Here's how the part is built. I have some questions about the finished solid (model axes, mm). A direction names the side the tool comes from. Round coordinates to 2 decimals unless told otherwise and drop trailing zeros. Write each loop counter-clockwise with the first axis right and the second up, starting at its lowest first coordinate (ties: lowest second). Pieces come first, ordered by that corner, then holes. Notation, with made-up numbers: (5, 21) -> (42, 21) arc R20 ccw to (42, 27) -> close; hole circle Ø9 at (-5.75, 65.25). An arc over 180 degrees is marked (long way). Put each result on its own line as item: value. Start each with the question number.
1) Will these pins go through, and if not, where does the flat tip stop? P1, Ø2.5, axis at x = -17.96, z = 17.96, coming from the +Y side; P2, Ø3, axis at y = 27, z = -2.5, coming from the +X side; P3, Ø17, axis at x = 11.5, y = 49, coming from the -Z side.
2) If I drill on line 1 along Y through (x, z) = (7, -7.5); line 2 along Z through (x, y) = (-21, 54); line 3 along X through (y, z) = (38, -17), over which ranges is the centre line in solid material (lowest first)? Write a range as [from, to].
3) I want a section at A-A, the plane y = 25. List the corners of the cut face in (x, z) for me.
4) I want a section at B-B, the plane z = -11. List the corners of the cut face in (x, y) for me.
5) I want a section at C-C, the plane z = 17. Give the number of separate pieces and of enclosed holes in the cut face, then the cut area to 3 significant figures.
6) We'd pull the mould along Z, two halves only. Please class faces 3 (the flat face through (-29, 64.77, 17)), 4 (the cylindrical face through (-19.169, 3.568, -19.856)), 5 (the flat face through (-15, 6, -29.21)), 6 (the cylindrical face through (16.752, 3.568, 16.065)): released by +Z, released by -Z, zero draft, split by the parting line, or undercut.
7) Which directions (+Z, -Z, +X, -X, +Y, -Y) give clear straight access to the entire face, cutting with the end or side of a thin tool? Please do faces 1 (the flat face through (0, 36, 29.21)), 2 (the cylindrical face through (16.752, 3.568, -19.856)).
from build123d import *

# Parameters (mm, degrees)
MOTORPROFILE_W                                    = 56
MOTORPROFILE_H                                    = 58.42
BOSS_EXTRUDE2_DEPTH                               = 8.89
BOSS_EXTRUDE3_DEPTH                               = 64.77
CSK_FOR_8_FLAT_HEAD_MACHINE_SCREW_100_D           = 4.4958
CSK_FOR_8_FLAT_HEAD_MACHINE_SCREW_100_CSINK_D     = 8.4328
CSK_FOR_8_FLAT_HEAD_MACHINE_SCREW_100_CSINK_ANGLE = 100


with BuildPart() as part:
    # MotorProfile → Boss-Extrude2 (new body)
    with BuildSketch(Plane(origin=(0, 0, 0), x_dir=(1, 0, 0), z_dir=(0, 1, 0))):
        Rectangle(MOTORPROFILE_W, MOTORPROFILE_H)
    extrude(amount=BOSS_EXTRUDE2_DEPTH)

    # Sketch2 → Boss-Extrude3 (add)
    with BuildSketch(Plane(origin=(0, 0, 0), x_dir=(1, 0, 0), z_dir=(0, 1, 0))):
        Polygon((-34.35, 29.21), (-34.35, -35.56), (28, -35.56), (28, -29.21), (-28, -29.21), (-28, 29.21), align=None)
    extrude(amount=BOSS_EXTRUDE3_DEPTH)

    # CSK for #8 Flat Head Machine Screw (100)2 (through all)
    with Locations(Plane(origin=(0, 8.89, 0), x_dir=(1, 0, 0), z_dir=(0, 1, 0))):
        with Locations((17.960512242, 17.960512242), (17.960512242, -17.960512242), (-17.960512242, -17.960512242), (-17.960512242, 17.960512242)):
            CounterSinkHole(CSK_FOR_8_FLAT_HEAD_MACHINE_SCREW_100_D / 2, CSK_FOR_8_FLAT_HEAD_MACHINE_SCREW_100_CSINK_D / 2, counter_sink_angle=CSK_FOR_8_FLAT_HEAD_MACHINE_SCREW_100_CSINK_ANGLE)


solid = part.part
Findings:
1. P1: passes through
1. P2: stops at x = -28
1. P3: stops at z = 29.21
2. line 1: y = [0, 8.89]
2. line 2: z = [29.21, 35.56]
2. line 3: x = [-34.35, -28]
3. outline: (-34.35, -29.21) -> (-28, -29.21) -> (-28, 29.21) -> (28, 29.21) -> (28, 35.56) -> (-34.35, 35.56) -> close
4. outline: (-34.35, 0) -> (28, 0) -> (28, 8.89) -> (-28, 8.89) -> (-28, 64.77) -> (-34.35, 64.77) -> close
5. separate pieces: 3
5. enclosed holes: 0
5. area: 830 mm2
6. face 3: zero draft
6. face 4: undercut
6. face 5: released by -Z
6. face 6: undercut
7. face 1: -Z, +X, +Y
7. face 2: +Y, -Y
